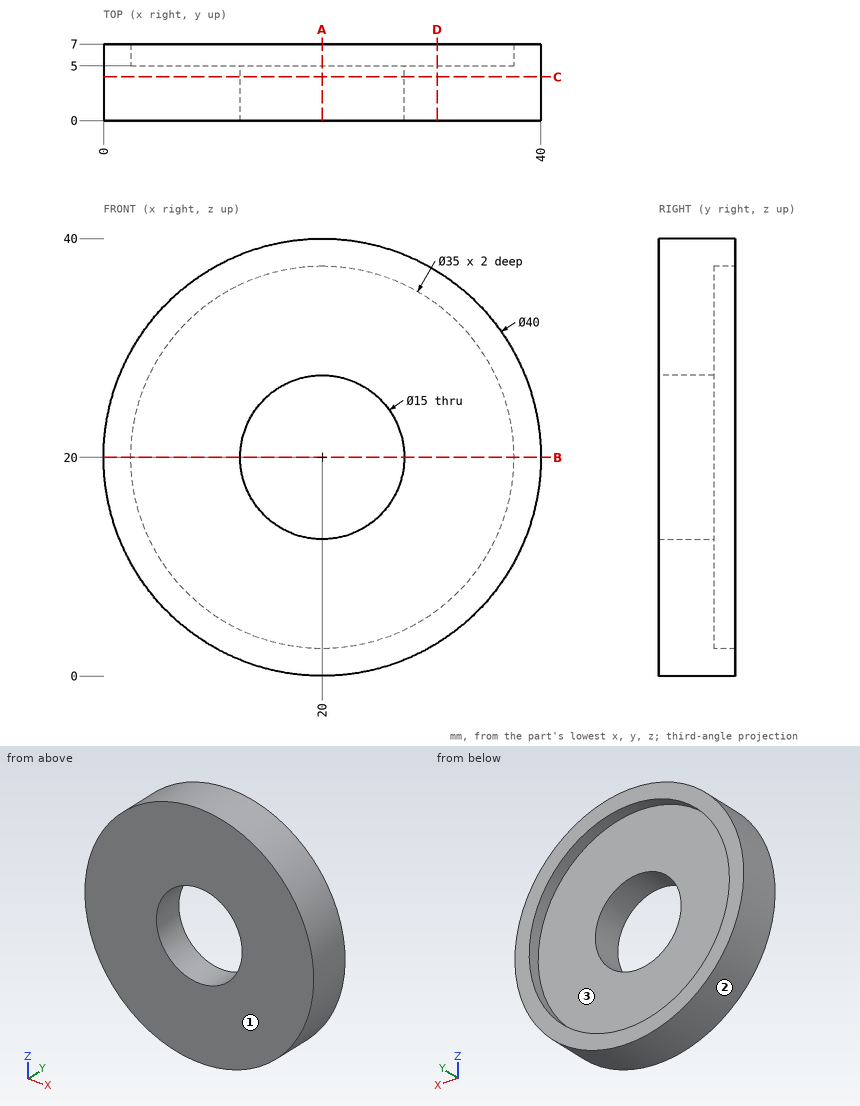
Design review of the part shown in the three views and the two pictorial views. Dimensions are in mm from the part's minimum x, y and z. Give positions to 0.01 mm unless a question says otherwise; leave off trailing zeros. Write each loop counter-clockwise with the first axis right and the second up, starting at its lowest first coordinate (ties: lowest second). Pieces come first, ordered by that corner, then holes. Notation, with made-up numbers: M 46,-33.75 L 101,-33.75 A7 ccw 101,-20.75 Z; hole C -12,21 d1. An arc over 180 degrees is marked long. Return JSON: item names as keys, results as strings. Group by question number.
Item 1: Take a section at D-D (x = 30.5). Give the boundary of the cut face in (y, z), plus the area to 3 significant figures.
Item 2: Take a section at C-C (y = 4). Give the boundary of the cut face in (x, z).
Item 3: The part is to be moulded in two halves that separate along Z. For the marked faces 1, 2 and 3, say which applies: pulls with the +Z half, pulls with the -Z half, needs draft (parallel to the pull), parting line crosses it, or undercut.
Item 4: Clearance check with flat-ended pins moving along their axes: pin 1 Ø10 at (x, z) = (20, 24) entering from +Y; pin 2 Ø4 at (y, z) = (1.5, 34.5) entering from +X; pin 3 Ø3 at (y, z) = (1.5, 36) entering from +X (3 decimals). State where each tip first meets the part, or that it passes through.
Item 5: Wall thickness on line 1 along X through (y, z) = (1.8, 20); line 2 along Y through (x, z) = (34.5, 28); line 3 along Z through (x, y) = (17.5, 6.5): over which ranges is each line inside the solid? List them lowest first.
Item 6: Take a section at B-B (z = 20). Give the boundary of the cut face in (x, y).
Item 7: Take a section at A-A (x = 20). Give the boundary of the cut face in (y, z).
Return value:
{
 "1": {"outline": "M 0,2.98 L 7,2.98 L 7,6 L 5,6 L 5,34 L 7,34 L 7,37.02 L 0,37.02 Z", "area": "182 mm2"},
 "2": {"outline": "C 20,20 d40; hole C 20,20 d15"},
 "3": {"face 1": "needs draft", "face 2": "parting line crosses it", "face 3": "undercut"},
 "4": {"pin 1": "stops at y = 5", "pin 2": "stops at x = 35.61", "pin 3": "stops at x = 33.775"},
 "5": {"line 1": "x = 0 to 12.5, 27.5 to 40", "line 2": "y = 0 to 5", "line 3": "z = 0.16 to 2.68, 37.32 to 39.84"},
 "6": {"outline": "M 0,0 L 12.5,0 L 12.5,5 L 2.5,5 L 2.5,7 L 0,7 Z; M 27.5,0 L 40,0 L 40,7 L 37.5,7 L 37.5,5 L 27.5,5 Z"},
 "7": {"outline": "M 0,0 L 7,0 L 7,2.5 L 5,2.5 L 5,12.5 L 0,12.5 Z; M 0,27.5 L 5,27.5 L 5,37.5 L 7,37.5 L 7,40 L 0,40 Z"}
}
